Can you work these out from the model? Positions are in its coordinate system, mm. Give positions to 0.01 mm unless a question says otherwise; leave off trailing zeros. Loops run counter-clockwise (first coordinate to the right, second up) from the corner with the lowest first, then second, coordinate; pieces in that order, holes last.
from build123d import *

# Parameters (mm, degrees)
F0_R     = 50
F1_DEPTH = 5


with BuildPart() as f1:
    # F0 (on Right) → F1 (new body)
    with BuildSketch(Plane.YZ):
        Circle(F0_R)
        with BuildLine():
            ThreePointArc((47.248112, 3.066945), (47.486037, 0.32898), (47.565433, -2.418156))
            ThreePointArc((47.565433, -2.418156), (47.565428, -2.440249), (47.565413, -2.462341))
            ThreePointArc((47.565413, -2.462341), (47.536276, -4.083355), (47.451912, -5.702434))
            ThreePointArc((47.451912, -5.702434), (47.241384, -7.960908), (46.923425, -10.206777))
            ThreePointArc((46.923425, -10.206777), (46.626401, -11.822901), (46.273731, -13.4278))
            ThreePointArc((46.273731, -13.4278), (45.790426, -15.290892), (45.232142, -17.132904))
            ThreePointArc((45.232142, -17.132904), (44.526808, -19.146391), (43.731895, -21.126225))
            ThreePointArc((43.731895, -21.126225), (42.925415, -22.909111), (42.046287, -24.657317))
            ThreePointArc((42.046287, -24.657317), (41.215832, -26.161064), (40.33162, -27.633844))
            ThreePointArc((40.33162, -27.633844), (39.257622, -29.275364), (38.116854, -30.871204))
            ThreePointArc((38.116854, -30.871204), (37.132326, -32.14459), (36.105277, -33.383935))
            ThreePointArc((36.105277, -33.383935), (0, -49.98359), (-36.105277, -33.383935))
            ThreePointArc((-36.105277, -33.383935), (-37.132326, -32.14459), (-38.116854, -30.871204))
            ThreePointArc((-38.116854, -30.871204), (-39.257622, -29.275364), (-40.33162, -27.633844))
            ThreePointArc((-40.33162, -27.633844), (-41.215832, -26.161064), (-42.046287, -24.657317))
            ThreePointArc((-42.046287, -24.657317), (-42.925415, -22.909111), (-43.731895, -21.126225))
            ThreePointArc((-43.731895, -21.126225), (-44.526808, -19.146391), (-45.232142, -17.132904))
            ThreePointArc((-45.232142, -17.132904), (-45.790426, -15.290892), (-46.273731, -13.4278))
            ThreePointArc((-46.273731, -13.4278), (-46.626401, -11.822901), (-46.923425, -10.206777))
            ThreePointArc((-46.923425, -10.206777), (-47.241384, -7.960908), (-47.451912, -5.702434))
            ThreePointArc((-47.451912, -5.702434), (-47.536276, -4.083355), (-47.565413, -2.462341))
            ThreePointArc((-47.565413, -2.462341), (-47.487308, 0.306924), (-47.248112, 3.066945))
            ThreePointArc((-47.248112, 3.066945), (-47.15882, 3.787982), (-47.058525, 4.507571))
            ThreePointArc((-47.058525, 4.507571), (-46.815862, 5.992878), (-46.526331, 7.469763))
            ThreePointArc((-46.526331, 7.469763), (-46.403436, 8.03132), (-46.273764, 8.591351))
            ThreePointArc((-46.273764, 8.591351), (-45.805713, 10.400077), (-45.266993, 12.189027))
            ThreePointArc((-45.266993, 12.189027), (-44.740599, 13.729576), (-44.161793, 15.251209))
            ThreePointArc((-44.161793, 15.251209), (-43.43838, 16.961669), (-42.648747, 18.642586))
            ThreePointArc((-42.648747, 18.642586), (-41.860885, 20.16805), (-41.018483, 21.664088))
            ThreePointArc((-41.018483, 21.664088), (-40.067748, 23.214753), (-39.05842, 24.727935))
            ThreePointArc((-39.05842, 24.727935), (-38.120143, 26.030484), (-37.138446, 27.30063))
            ThreePointArc((-37.138446, 27.30063), (-35.80078, 28.899165), (-34.394365, 30.43756))
            ThreePointArc((-34.394365, 30.43756), (-33.212951, 31.631371), (-31.990127, 32.782727))
            ThreePointArc((-31.990127, 32.782727), (-30.127888, 34.389191), (-28.185102, 35.897252))
            ThreePointArc((-28.185102, 35.897252), (-26.603538, 37.011809), (-24.977955, 38.061125))
            ThreePointArc((-24.977955, 38.061125), (0, 45.147277), (24.977955, 38.061125))
            ThreePointArc((24.977955, 38.061125), (26.603538, 37.011809), (28.185102, 35.897252))
            ThreePointArc((28.185102, 35.897252), (30.127888, 34.389191), (31.990127, 32.782727))
            ThreePointArc((31.990127, 32.782727), (33.212951, 31.631371), (34.394365, 30.43756))
            ThreePointArc((34.394365, 30.43756), (35.80078, 28.899165), (37.138446, 27.30063))
            ThreePointArc((37.138446, 27.30063), (38.120143, 26.030484), (39.05842, 24.727935))
            ThreePointArc((39.05842, 24.727935), (40.067748, 23.214753), (41.018483, 21.664088))
            ThreePointArc((41.018483, 21.664088), (41.860885, 20.16805), (42.648747, 18.642586))
            ThreePointArc((42.648747, 18.642586), (43.43838, 16.961669), (44.161793, 15.251209))
            ThreePointArc((44.161793, 15.251209), (44.740599, 13.729576), (45.266993, 12.189027))
            ThreePointArc((45.266993, 12.189027), (45.805713, 10.400077), (46.273764, 8.591351))
            ThreePointArc((46.273764, 8.591351), (46.403436, 8.03132), (46.526331, 7.469763))
            ThreePointArc((46.526331, 7.469763), (46.815862, 5.992878), (47.058525, 4.507571))
            ThreePointArc((47.058525, 4.507571), (47.15882, 3.787982), (47.248112, 3.066945))
        make_face(mode=Mode.SUBTRACT)
    extrude(amount=F1_DEPTH)


solid = f1.part
(1) Suppose I cut it at B-B on z = -15. List the corners of the cut face in (x, y) for me, plus the area to 3 significant figures.
Returned:
outline: (0, -47.7) - (5, -47.7) - (5, -45.87) - (0, -45.87) - close; (0, 45.87) - (5, 45.87) - (5, 47.7) - (0, 47.7) - close
area: 18.3 mm2
(2) Will these pins go through, and if not, where does the flat tip stop? P1, Ø1, axis at x = 2.5, z = 21.5, coming from the +Y side; P2, Ø1.5, axis at y = -31.5, z = 38.5, coming from the -X side; P3, Ø1.5, axis at x = 3.5, y = 18, coming from the -Z side.
Returned:
P1: stops at y = 45.38
P2: stops at x = 0
P3: stops at z = -46.93
(3) Please list where these lines run through material, in increasing order: probe 1 along Z at (x, y) = (4.7, -18.5); probe 2 along Z at (x, y) = (1.4, -40); probe 3 along Y at (x, z) = (3.65, -19).
Returned:
probe 1: z = -46.45 to -46.24, 41.4 to 46.45
probe 2: z = -30 to -28.16, 23.32 to 30
probe 3: y = -46.25 to -44.58, 44.58 to 46.25
(4) Thinking about a two-plate mould opening in Y: for faces 1 (the cylindrical face through (2.465, 47.484, 0.367)), 2 (the flat face through (5, 7, 45)), which applies, pulls with the +Y half, pulls with the -Y half, needs draft (parallel to the pull), parting line crosses it, or undercut?
Returned:
face 1: undercut
face 2: needs draft
